Check sheet for the modelled part. Datum: model origin and axes. Units: mm. A direction names the side the tool comes from. Round coordinates to 2 decimals unless told otherwise and drop trailing zeros. Write each loop counter-clockwise with the first axis right and the second up, starting at its lowest first coordinate (ties: lowest second). Pieces come first, ordered by that corner, then holes. Notation, with made-up numbers: (75.5, -13) -> (131.5, -13) arc R19 ccw to (131.5, -4) -> close; hole circle Ø11 at (69, 34.5). An arc over 180 degrees is marked (long way). One line per item, written item: value.
Autodesk Inventor part; units mm, degrees
ref_plane "YZ Plane" through (0, 0, 0) normal (1, 0, 0) x (0, 1, 0)
ref_plane "XZ Plane" through (0, 0, 0) normal (0, 1, 0) x (-1, 0, 0)
ref_plane "XY Plane" through (0, 0, 0) normal (0, 0, 1) x (1, 0, 0)
sketch "Sketch1" plane through (0, 0, 0) normal (1, 0, 0) x (0, 1, 0)
  line L0 (0, 0) -> (20, 0)
  line L1 (20, 0) -> (0, -19)
  line L2 (0, -19) -> (0, 0)
  dimension "d0" = 20
  dimension "d1" = 19
extrude "Extrusion1" add sketch "Sketch1" along normal blind 40
sketch "Sketch2" plane through (0, 0, -19) normal (0, -1, 0) x (1, 0, 0)
  line L0 (40, 19) -> (40, 0)
  line L1 (40, 0) -> (0, 0)
  line L2 (0, 0) -> (0, 5)
  line L3 (0, 5) -> (40, 5)
  line L4 (40, 5) -> (40, 0)
  point P0 (0, 19)
  dimension "d4" = 5
extrude "Extrusion2" add sketch "Sketch2" along normal blind 11.5
sketch "Sketch3" plane through (0, 0, -14) normal (0, 0, 1) x (1, 0, 0)
  line L0 (40, 0) -> (40, -11.5)
  line L1 (0, -11.5) -> (40, -11.5)
  line L2 (40, -11.5) -> (40, -6.5)
  line L3 (40, -6.5) -> (0, -6.5)
  line L4 (0, -6.5) -> (0, -11.5)
  point P0 (0, 0)
  dimension "d7" = 5
extrude "Extrusion3" add sketch "Sketch3" along normal blind 14
properties part number "Ooze_Ramp_Bottom"
Item 1: Release check for a two-part mould opening along Y. For faces 3 (the flat face through (20, 10, 0)), 4 (the flat face through (20, -3, -14)), 5 (the flat face through (19.72, 10.14, -9.367)) record: pulls with the +Y half, pulls with the -Y half, needs draft (parallel to the pull), parting line crosses it, or undercut.
Result set:
face 3: needs draft
face 4: undercut
face 5: pulls with the +Y half
Item 2: Sectioned sample at C-C (y = 4). Enter the section's corners in (x, z), then the cut area to 3 significant figures.
Result set:
outline: (0, -15.2) -> (40, -15.2) -> (40, 0) -> (0, 0) -> close
area: 608 mm^2
Item 3: Sectioned sample at A-A (x = 12). Enter the section's corners in (y, z), then the cut area to 4 significant figures.
Result set:
outline: (-11.5, -19) -> (0, -19) -> (20, 0) -> (0, 0) -> (0, -14) -> (-6.5, -14) -> (-6.5, 0) -> (-11.5, 0) -> close
area: 317.5 mm^2
Item 4: Depth check by flat-ended pin: pin 1 (4 mm diameter, centred on x = 17.5, z = -10, fed in from +Y); pin 2 (3 mm diameter, centred on x = 5.5, y = 5.5, fed in from +Z); pin 3 (2 mm diameter, centred on x = 14.5, y = -4, fed in from +Z); pin 4 (3 mm diameter, centred on x = 29, z = -10, fed in from +Y). Enter the tip coordinate at first touch or a pass-through.
Result set:
pin 1: y = 11.58
pin 2: z = 0
pin 3: z = -14
pin 4: y = 11.05
Item 5: Tool access check on faces 1 (the flat face through (20, -6.5, -7)), 2 (the flat face through (20, -9, 0)). Record the directions out of +Z, -Z, +X, -X, +Y, -Y that give a thin tool (end or side, any length) a straight path to the whole face; none if there is none.
Result set:
face 1: +Z, +X, -X
face 2: +Z, +X, -X, +Y, -Y
Item 6: Sectioned sample at D-D (z = -11.5). Enter the section's corners in (x, y).
Result set:
outline: (0, -11.5) -> (40, -11.5) -> (40, -6.5) -> (0, -6.5) -> close; (0, 0) -> (40, 0) -> (40, 7.89) -> (0, 7.89) -> close
Item 7: Material ranges on line 1 along Y through (x, z) = (10.5, -2); line 2 along Z through (x, y) = (23, -3); line 3 along Y through (x, z) = (18.5, -7), recorded low to high.
Result set:
line 1: -11.5 to -6.5, 0 to 17.89
line 2: -19 to -14
line 3: -11.5 to -6.5, 0 to 12.63
Item 8: Sectioned sample at B-B (z = -8.75). Enter the section's corners in (x, y), then the cut area to 3 significant figures.
Result set:
outline: (0, -11.5) -> (40, -11.5) -> (40, -6.5) -> (0, -6.5) -> close; (0, 0) -> (40, 0) -> (40, 10.79) -> (0, 10.79) -> close
area: 632 mm^2
